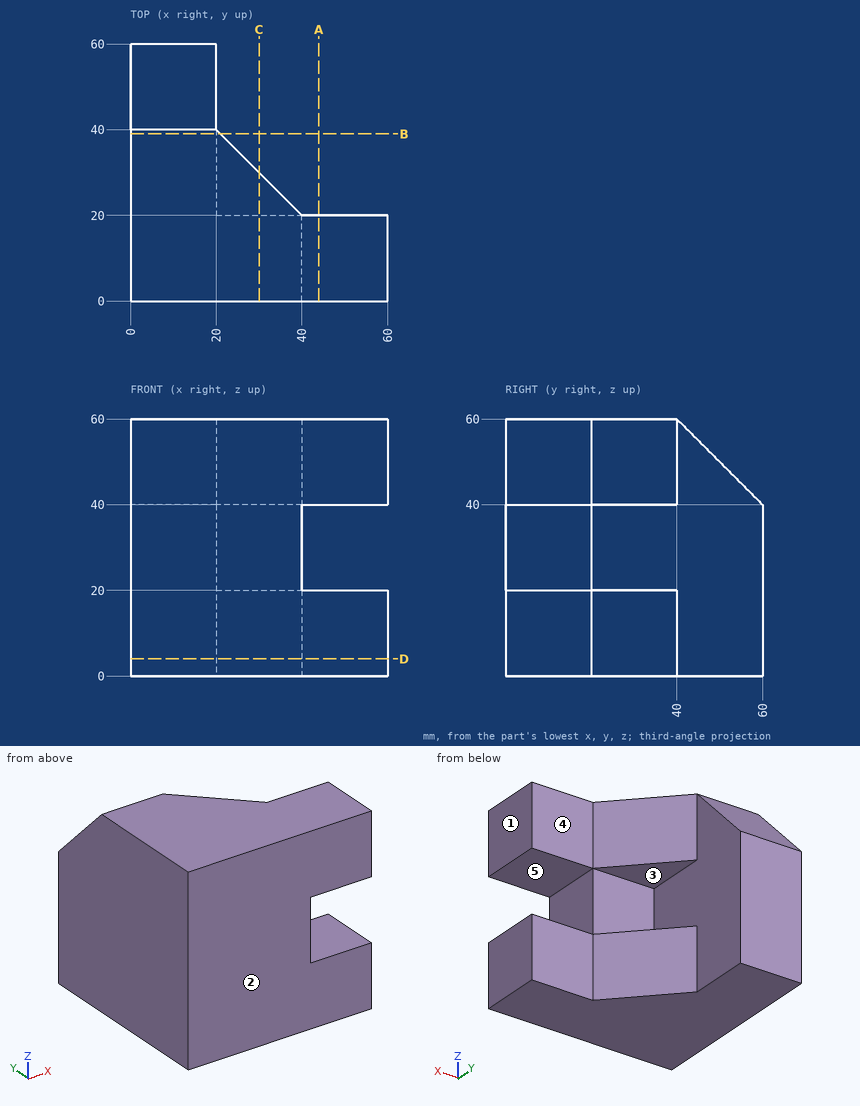
Could you check a few things on this drawing? It's one solid part, dimensions in mm from its lowest x, y, z. A direction names the side the tool comes from. Give positions to 0.01 mm unless a question says otherwise; leave off trailing zeros. Loops run counter-clockwise (first coordinate to the right, second up) from the corner with the lowest first, then second, coordinate; pieces in that order, holes last. Notation, with made-up numbers: (-6, 87.5) -> (47, 87.5) arc R23 cw to (47, 103.5) -> close; hole circle Ø10 at (68, -33). An arc over 180 degrees is marked (long way). Answer as CSV lines item,"result". Start each with the question number.
(1) I'm going to push flat-ended pins straight in: pin 1 Ø16 at (x, z) = (29, 28.5) entering from +Y; pin 2 Ø1.5 at (y, z) = (30.5, 53) entering from +X; pin 3 Ø16 at (x, z) = (46.5, 51.5) entering from +Y. Where does each tip first touch, or does it pass through?
(2) If we section it at A-A on x = 44: Write out the boundary of the cut face in (y, z), then the cut area to 3 significant figures.
(3) If we section it at D-D on z = 4: Write out the boundary of the cut face in (x, y), then the cut area to 3 significant figures.
(4) Which directions (+Z, -Z, +X, -X, +Y, -Y) give clear straight access to the entire face, cutting with the end or side of a thin tool? Please do the marked faces 1, 2, 3, 4 and 5.
(5) I need wall thicknesses on probe 1 along X at (y, z) = (4, 28.5); probe 2 along X at (y, z) = (45, 27.5); probe 3 along Z at (x, y) = (25, 22). Which ranges of each line are inside material? Lowest first, please.
(6) If we section it at C-C on x = 30: Write out the boundary of the cut face in (y, z).
(7) If we section it at B-B on y = 39: Write out the boundary of the cut face in (x, z).
Computed:
1,pin 1,"stops at y = 20"
1,pin 2,"stops at x = 30.25"
1,pin 3,"stops at y = 21.5"
2,outline,"(0, 0) -> (20, 0) -> (20, 20) -> (0, 20) -> close; (0, 40) -> (20, 40) -> (20, 60) -> (0, 60) -> close"
2,area,"800 mm2"
3,outline,"(0, 0) -> (60, 0) -> (60, 20) -> (40, 20) -> (20, 40) -> (20, 60) -> (0, 60) -> close"
3,area,"2,200 mm2"
4,face 1,"+Z, -Z, +X, +Y, -Y"
4,face 2,"+Z, -Z, +X, -X, -Y"
4,face 3,"+X, +Y"
4,face 4,"+Z, -Z, +X, +Y"
4,face 5,"+X, +Y, -Y"
5,probe 1,"x = 0 to 40"
5,probe 2,"x = 0 to 20"
5,probe 3,"z = 0 to 20, 40 to 60"
6,outline,"(0, 0) -> (30, 0) -> (30, 20) -> (20, 20) -> (20, 40) -> (30, 40) -> (30, 60) -> (0, 60) -> close"
7,outline,"(0, 0) -> (21, 0) -> (21, 20) -> (20, 20) -> (20, 40) -> (21, 40) -> (21, 60) -> (0, 60) -> close"
